The listing builds one solid part. Answer for the finished solid, in the listing's coordinates (mm). A direction names the side the tool comes from. Coordinates: 2 decimals unless noted, no trailing zeros. Order: outer loops, then holes, each group sorted by start corner. A loop starts at its lowest first (then second) coordinate and runs counter-clockwise, first axis right, second up.
```python
from build123d import *

# Parameters (mm, degrees)
SKETCH1_R           = 34
SKETCH1_R_2         = 32
BOSS_EXTRUDE1_DEPTH = 12
SKETCH1_2_R         = 34
SKETCH1_2_R_2       = 32
BOSS_EXTRUDE2_DEPTH = 12
SKETCH1_3_R         = 32
BOSS_EXTRUDE3_DEPTH = 2


with BuildPart() as part:
    # Sketch1 → Boss-Extrude1 (new body)
    with BuildSketch(Plane(origin=(0, 0, 0), x_dir=(1, 0, 0), z_dir=(0, 1, 0))):
        with Locations(Location((0, 0, 0), (0, 0, 270))):
            Circle(SKETCH1_R)
        with Locations(Location((0, 0, 0), (0, 0, 270))):
            Circle(SKETCH1_R_2, mode=Mode.SUBTRACT)
    extrude(amount=BOSS_EXTRUDE1_DEPTH)

    # Sketch1_2 → Boss-Extrude2 (add)
    with BuildSketch(Plane(origin=(0, 0, 0), x_dir=(1, 0, 0), z_dir=(0, 1, 0))):
        with Locations(Location((0, 0, 0), (0, 0, 270))):
            Circle(SKETCH1_2_R)
        with Locations(Location((0, 0, 0), (0, 0, 270))):
            Circle(SKETCH1_2_R_2, mode=Mode.SUBTRACT)
    extrude(amount=BOSS_EXTRUDE2_DEPTH)

    # Sketch1_3 → Boss-Extrude3 (add)
    with BuildSketch(Plane(origin=(0, 0, 0), x_dir=(1, 0, 0), z_dir=(0, 1, 0))):
        with Locations(Location((0, 0, 0), (0, 0, 270))):
            Circle(SKETCH1_3_R)
    extrude(amount=BOSS_EXTRUDE3_DEPTH)


solid = part.part
```
1) A cutting plane is placed at A-A, the plane x = 0. Write down the section's boundary in (y, z), plus the area to 3 significant figures.
2) Straight lines are drawn through the part: probe 1 along Y at (x, z) = (4.5, 29); probe 2 along X at (y, z) = (6, 0); probe 3 along X at (y, z) = (11, -3.5). For each, find the intervals that lie inside material, in ascending order.
3) Each of these flat-tipped pins is pushed along its axis until it touches: P1, Ø12, axis at x = -6.5, z = 25, coming from the +Y side; P2, Ø1.5, axis at y = 8.5, z = 17, coming from the -X side; P3, Ø5, axis at y = 9.5, z = 12.5, coming from the +X side. Where does it stop, or does it pass through?
4) A cutting plane is placed at C-C, the plane y = 9.25. Write down the section's boundary in (x, z).
5) The mould has two halves that part along X. Classify faces 3 (the cylindrical face through (33.71, 5.92, -4.43)), 4 (the flat face through (0, 2, 0)), 5 (the flat face through (0, 0, 0)): released by +X, released by -X, zero draft, split by the parting line, or undercut.
6) A cutting plane is placed at B-B, the plane z = 18.5. Write down the section's boundary in (x, y), plus the area to 3 significant figures.
7) For faces 1 (the cylindrical face through (-31.24, 6.93, -6.94)), 2 (the flat face through (-23, 12, -23)), determine the directions among +Z, -Z, +X, -X, +Y, -Y from which every point of the face is accessible in a straight line to the end or side of a thin tool.
Working result:
1. outline: (0, -34) - (12, -34) - (12, -32) - (2, -32) - (2, 32) - (12, 32) - (12, 34) - (0, 34) - close
1. area: 176 mm2
2. probe 1: y = 0 to 2
2. probe 2: x = -34 to -32, 32 to 34
2. probe 3: x = -33.82 to -31.81, 31.81 to 33.82
3. P1: stops at y = 2
3. P2: stops at x = -29.87
3. P3: stops at x = 32.5
4. outline: circle Ø68 at (0, 0); hole circle Ø64 at (0, 0)
5. face 3: split by the parting line
5. face 4: undercut
5. face 5: zero draft
6. outline: (-28.53, 0) - (28.53, 0) - (28.53, 12) - (26.11, 12) - (26.11, 2) - (-26.11, 2) - (-26.11, 12) - (-28.53, 12) - close
6. area: 162 mm2
7. face 1: +Y
7. face 2: +Z, -Z, +X, -X, +Y
